Could you check a few things on this drawing? It's one solid part, dimensions in mm from its lowest x, y, z. Round coordinates to 2 decimals unless told otherwise and drop trailing zeros. Loops run counter-clockwise (first coordinate to the right, second up) from the corner with the lowest first, then second, coordinate; pieces in that order, holes last. Notation, with made-up numbers: (61.25, 50) -> (108.25, 50) arc R34 cw to (108.25, 86) -> close; hole circle Ø7 at (-37.75, 22.5). An arc over 180 degrees is marked (long way). Put each result on its own line as item: value. Start each with the question number.
1. I need wall thicknesses on line 1 (Y direction, x = 30, z = 2.75); line 2 (Y direction, x = 530, z = 2) (1 decimal); line 3 (Y direction, x = 663.5, z = 7.75) (1 decimal). Which ranges of each line are inside material? Lowest first, please. Write a range as [from, to].
2. Imagine slicing it at C-C, the plane y = 432.5. Please give me the cut outline in (x, z), and give its area (3 significant figures).
3. Imagine slicing it at D-D, the plane x = 88. Please give me the cut outline in (y, z), and give its area (3 significant figures).
4. Imagine slicing it at A-A, the plane z = 4.25. Please give me the cut outline in (x, y).
5. I'm going to push flat-ended pins straight in: P1, Ø4, axis at y = 284, z = 2, coming from the +X side; P2, Ø1.5, axis at y = 161.5, z = 8.5, coming from the +X side. Where does each tip first touch, or does it pass through?
6. Imagine slicing it at B-B, the plane x = 530. Please give me the cut outline in (y, z) (1 decimal).
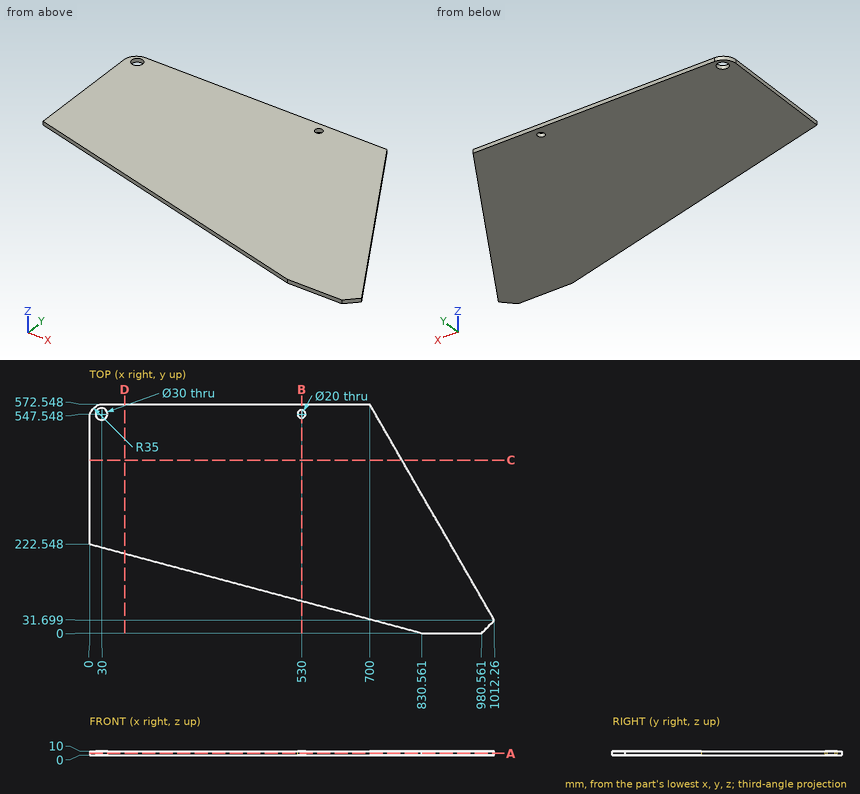
Entries:
1. line 1: [214.51, 532.55], [562.55, 572.19]
1. line 2: [80.5, 537.5], [557.5, 572.5]
1. line 3: [44.8, 572.5]
2. outline: (0, 0) -> (780.86, 0) -> (780.86, 10) -> (0, 10) -> close
2. area: 7,810 mm^2
3. outline: (198.97, 0) -> (572.55, 0) -> (572.55, 10) -> (198.97, 10) -> close
3. area: 3,740 mm^2
4. outline: (0, 222.55) -> (830.56, 0) -> (980.56, 0) -> (1012.26, 31.7) -> (700, 572.55) -> (35, 572.55) arc R35 ccw to (0, 537.55) -> close; hole circle Ø30 at (30, 547.55); hole circle Ø20 at (530, 547.55)
5. P1: x = 867.75
5. P2: x = 937.75
6. outline: (80.5, 0) -> (537.5, 0) -> (537.5, 10) -> (80.5, 10) -> close; (557.5, 0) -> (572.5, 0) -> (572.5, 10) -> (557.5, 10) -> close
